```python
from build123d import *

# Parameters (mm, degrees)
F0_W     = 304.8
F0_H     = 12.7
F1_DEPTH = 406.4
F3_D     = 7.9375
F3_DEPTH = 20.6629
F3_TIP   = 2.3846655818
F4_D     = 10.0838
F4_DEPTH = 20.6756
F4_TIP   = 3.0294791551
F5_D     = 16.66748
F5_DEPTH = 19.1008
F5_TIP   = 5.0074161752
F7_D     = 3.7973
F7_DEPTH = 19.1008
F7_TIP   = 1.1408240143


with BuildPart() as f1:
    # F0 (on Front) → F1 (new body)
    with BuildSketch(Plane.XZ):
        with Locations((152.4, 6.35)):
            Rectangle(F0_W, F0_H)
    extrude(amount=F1_DEPTH)

    # F3
    with Locations(Plane.XY.offset(12.7)):
        with Locations((41.275, -381), (41.275, -203.2), (41.275, -25.4), (263.525, -25.4), (263.525, -203.2), (263.525, -381)):
            Hole(F3_D / 2, depth=F3_DEPTH)
            with Locations((0, 0, -(F3_DEPTH + F3_TIP / 2))):  # 118° drill point
                Cone(0, F3_D / 2, F3_TIP, mode=Mode.SUBTRACT)

    # F4
    with Locations(Plane.XY.offset(12.7)):
        with Locations((73.025, -381), (73.025, -203.2), (73.025, -25.4), (231.775, -381), (231.775, -203.2), (231.775, -25.4)):
            Hole(F4_D / 2, depth=F4_DEPTH)
            with Locations((0, 0, -(F4_DEPTH + F4_TIP / 2))):  # 118° drill point
                Cone(0, F4_D / 2, F4_TIP, mode=Mode.SUBTRACT)

    # F5
    with Locations(Plane.XY.offset(12.7)):
        with Locations((152.4, -203.2)):
            Hole(F5_D / 2, depth=F5_DEPTH)
            with Locations((0, 0, -(F5_DEPTH + F5_TIP / 2))):  # 118° drill point
                Cone(0, F5_D / 2, F5_TIP, mode=Mode.SUBTRACT)

    # F7
    with Locations(Plane.XY.offset(12.7)):
        with Locations((28.575, -31.75), (276.225, -31.75), (276.225, -146.05), (276.225, -260.35), (276.225, -374.65), (28.575, -374.65), (28.575, -260.35), (28.575, -146.05)):
            Hole(F7_D / 2, depth=F7_DEPTH)
            with Locations((0, 0, -(F7_DEPTH + F7_TIP / 2))):  # 118° drill point
                Cone(0, F7_D / 2, F7_TIP, mode=Mode.SUBTRACT)


solid = f1.part
```
Can you work these out from the model? Positions are in its coordinate system, mm. Give positions to 0.01 mm unless a question says otherwise; leave off trailing zeros. Loops run counter-clockwise (first coordinate to the right, second up) from the corner with the lowest first, then second, coordinate; pieces in that order, holes last. Notation, with made-up numbers: M -23,36 L 31,36 A6 ccw 31,46 Z; hole C 35,27.25 d9. An arc over 180 degrees is marked long. Use one line per item in the form item = value. Start each with the question number.
(1) I want a section at A-A, the plane x = 153. Write out the boundary of the cut face in (y, z).
(2) I'm going to push flat-ended pins straight in: P1, Ø5, axis at x = 263.525, y = -203.2, coming from the +Z side; P2, Ø16, axis at x = 231.775, y = -203.2, coming from the +Z side. Where does each tip first touch, or does it pass through?
(3) Thinking about a two-plate mould opening in Y: for faces 1 (the flat face through (150, 0, 6)), 2 (the cylindrical face through (74.12, -208.12, 6.26)), 3 (the flat face through (184, -200, 0)), which applies, released by +Y, released by -Y, zero draft, split by the parting line, or undercut?
(4) Please list where these lines run through material, in increasing order: line 1 (X direction, y = -260.35, z = 8.5); line 2 (Y direction, x = 75, z = 2); line 3 (Y direction, x = 152.4, z = 4.5).
Worked out:
q1.outline = M -406.4,0 L -211.51,0 L -211.51,12.7 L -406.4,12.7 Z; M -194.89,0 L 0,0 L 0,12.7 L -194.89,12.7 Z
q2.P1 = through
q2.P2 = 12.7
q3.face_1 = released by +Y
q3.face_2 = undercut
q3.face_3 = zero draft
q4.line_1 = 0 to 26.68, 30.47 to 274.33, 278.12 to 304.8
q4.line_2 = -406.4 to -385.64, -376.36 to -207.84, -198.56 to -30.04, -20.76 to 0
q4.line_3 = -406.4 to -211.53, -194.87 to 0
